from build123d import *

# Parameters (mm, degrees)
ESQUISSE2_W             = 5
ESQUISSE2_H             = 12.5
ESQUISSE3_R             = 2
ENL_V_MAT_EXTRU_1_DEPTH = 36
ESQUISSE4_R             = 3.5
ENL_V_MAT_EXTRU_2_DEPTH = 36
SKETCH1_R               = 40
CUT_EXTRUDE1_DEPTH      = 20
SKETCH2_R               = 40
SKETCH2_R_2             = 39
BOSS_EXTRUDE2_DEPTH     = 15
SKETCH3_R               = 25
CUT_EXTRUDE2_DEPTH      = 5
SKETCH4_R               = 43.5
SKETCH4_R_2             = 40
BOSS_EXTRUDE3_DEPTH     = 20
SKETCH5_R               = 43.5
SKETCH5_R_2             = 40.45
CUT_EXTRUDE3_DEPTH      = 1.55
SKETCH6_R               = 43.5
SKETCH6_R_2             = 40.45
CUT_EXTRUDE4_DEPTH      = 1.55
CUT_EXTRUDE4_DEPTH_BACK = 1.55
SKETCH7_R               = 43.5
SKETCH7_R_2             = 40.45
CUT_EXTRUDE5_DEPTH      = 1.55


with BuildPart() as part:
    # Esquisse1 → Révolution1 (revolve)
    with BuildSketch(Plane.XY):
        Polygon((0, 34), (0, 0), (8, 0), (8, 40), (3, 40), (3, 39), (-27, 39), (-27, 40), (-32, 40), (-32, 34), align=None)
    revolve(axis=Axis((-49.644499027, 0, 0), (1, 0, 0)))

    # Esquisse2 → Enlèvement de matière-Révolution1 (revolve, cut)
    with BuildSketch(Plane.XY):
        with Locations((5.5, 6.25)):
            Rectangle(ESQUISSE2_W, ESQUISSE2_H)
    revolve(axis=Axis((0, 0, 0), (1, 0, 0)), mode=Mode.SUBTRACT)

    # Esquisse3 → Enlèv. mat.-Extru.1 (cut, through all)
    with BuildSketch(Plane(origin=(3, 0, 0), x_dir=(0, 0, -1), z_dir=(1, 0, 0))):
        with Locations((4.75, 8.227241336)):
            Circle(ESQUISSE3_R)
        with Locations((-4.75, 8.227241336)):
            Circle(ESQUISSE3_R)
        with Locations((4.75, -8.227241336)):
            Circle(ESQUISSE3_R)
        with Locations((-4.75, -8.227241336)):
            Circle(ESQUISSE3_R)
    extrude(amount=-ENL_V_MAT_EXTRU_1_DEPTH, mode=Mode.SUBTRACT)

    # Esquisse4 → Enlèv. mat.-Extru.2 (cut, through all)
    with BuildSketch(Plane(origin=(3, 0, 0), x_dir=(0, 0, -1), z_dir=(1, 0, 0))):
        Circle(ESQUISSE4_R)
    extrude(amount=-ENL_V_MAT_EXTRU_2_DEPTH, mode=Mode.SUBTRACT)

    # Sketch1 → Cut-Extrude1 (cut)
    with BuildSketch(Plane.ZY.offset(32)):
        Circle(SKETCH1_R)
    extrude(amount=-CUT_EXTRUDE1_DEPTH, mode=Mode.SUBTRACT)

    # Sketch2 → Boss-Extrude2 (add)
    with BuildSketch(Plane.ZY.offset(-3)):
        Circle(SKETCH2_R)
        Circle(SKETCH2_R_2, mode=Mode.SUBTRACT)
    extrude(amount=BOSS_EXTRUDE2_DEPTH)

    # Sketch3 → Cut-Extrude2 (cut)
    with BuildSketch(Plane(origin=(8, 0, 0), x_dir=(0, 0, -1), z_dir=(1, 0, 0))):
        Circle(SKETCH3_R)
    extrude(amount=-CUT_EXTRUDE2_DEPTH, mode=Mode.SUBTRACT)

    # Sketch4 → Boss-Extrude3 (add)
    with BuildSketch(Plane.ZY.offset(12)):
        Circle(SKETCH4_R)
        Circle(SKETCH4_R_2, mode=Mode.SUBTRACT)
    extrude(amount=-BOSS_EXTRUDE3_DEPTH)

    # Sketch5 → Cut-Extrude3 (cut)
    with BuildSketch(Plane.ZY.offset(12)):
        Circle(SKETCH5_R)
        Circle(SKETCH5_R_2, mode=Mode.SUBTRACT)
    extrude(amount=-CUT_EXTRUDE3_DEPTH, mode=Mode.SUBTRACT)

    # Sketch6 → Cut-Extrude4 (cut, two sides)
    with BuildSketch(Plane.ZY.offset(2)) as cut_extrude4_sk:
        Circle(SKETCH6_R)
        Circle(SKETCH6_R_2, mode=Mode.SUBTRACT)
    extrude(amount=CUT_EXTRUDE4_DEPTH, mode=Mode.SUBTRACT)
    extrude(cut_extrude4_sk.sketch, amount=-CUT_EXTRUDE4_DEPTH_BACK, mode=Mode.SUBTRACT)

    # Sketch7 → Cut-Extrude5 (cut)
    with BuildSketch(Plane(origin=(8, 0, 0), x_dir=(0, 0, -1), z_dir=(1, 0, 0))):
        Circle(SKETCH7_R)
        Circle(SKETCH7_R_2, mode=Mode.SUBTRACT)
    extrude(amount=-CUT_EXTRUDE5_DEPTH, mode=Mode.SUBTRACT)


solid = part.part
Input: part model. Units: mm. Frame: model coordinates. A direction names the side the tool comes from. Give positions to 0.01 mm unless a question says otherwise; leave off trailing zeros. Order: outer loops, then holes, each group sorted by start corner. A loop starts at its lowest first (then second) coordinate and runs counter-clockwise, first axis right, second up.
Q1. Set-up query: faces 1 (the cylindrical face through (5.535, 7.509, -23.846)), 2 (the cylindrical face through (-5.92, 18.28, 28.67)), 3 (the cylindrical face through (2.95, 43.13, -5.66)), 4 (the flat face through (-0.45, -29, 29)). Return all of +Z, -Z, +X, -X, +Y, -Y with unobstructed straight access to the full face (end or side cutting, diameter ignored); none if empty.
Checked values:
face 1: +X
face 2: -X
face 3: +X, -X
face 4: none
Q2. Draft query along Y for faces 5 (the cylindrical face through (1.521, -1.341, -3.233)), 6 (the flat face through (6.45, -29, -29)), 7 (the cylindrical face through (-7.05, 43.13, -5.66)). Return one class per face: +Y half, -Y half, draft (parallel to the pull), parting line (faces both ways), or undercut.
Checked values:
face 5: undercut
face 6: draft
face 7: parting line
Q3. Contact query for flat-ended pins moving along their axis: pin 1 Ø1 at (x, y) = (-0.5, 11.5) entering from +Z; pin 2 Ø3.5 at (y, z) = (-8.23, -4.75) entering from +X; pin 3 Ø4 at (x, z) = (-4.5, -30.5) entering from +Y; pin 4 Ø8 at (x, z) = (-6, 32.5) entering from -Y. Output: stop coordinate, or through.
Checked values:
pin 1: stops at z = 42.09
pin 2: passes through
pin 3: stops at y = 32.86
pin 4: stops at y = -32.86
Q4. Section D-D on x = -6. Output: boundary loops of the cut face in (y, z).
Checked values:
outline: circle Ø87 at (0, 0); hole circle Ø68 at (0, 0)
Q5. Section C-C on z = 18.5. Output: boundary loops of the cut face in (x, y).
Checked values:
outline: (-12, -35.97) - (-10.45, -35.97) - (-10.45, -39.37) - (-3.55, -39.37) - (-3.55, -35.97) - (-0.45, -35.97) - (-0.45, -39.37) - (6.45, -39.37) - (6.45, -35.97) - (8, -35.97) - (8, -16.82) - (3, -16.82) - (3, 16.82) - (8, 16.82) - (8, 35.97) - (6.45, 35.97) - (6.45, 39.37) - (-0.45, 39.37) - (-0.45, 35.97) - (-3.55, 35.97) - (-3.55, 39.37) - (-10.45, 39.37) - (-10.45, 35.97) - (-12, 35.97) - (-12, 28.53) - (0, 28.53) - (0, -28.53) - (-12, -28.53) - close
Q6. Ray query, probe 1 along Y at (x, z) = (0.95, 0); probe 2 along X at (y, z) = (1, 32); probe 3 along X at (y, z) = (-14, 19). Return the intervals inside material, ascending.
Checked values:
probe 1: y = -43.5 to -3.5, 3.5 to 43.5
probe 2: x = 0 to 8
probe 3: x = 0 to 3
